Could you check a few things on this model? Use its own coordinates, in mm. A direction names the side the tool comes from. Give positions to 0.01 mm unless a question says otherwise; leave off trailing zeros. Loops run counter-clockwise (first coordinate to the right, second up) from the corner with the lowest first, then second, coordinate; pieces in that order, holes last. Notation, with made-up numbers: (-28.75, 6) -> (6.25, 6) arc R21 ccw to (6.25, 30) -> close; hole circle Ø11 at (-16.75, -19.5). An arc over 180 degrees is marked (long way). Write item = value, one per line. Start each with the question number.
1) I need wall thicknesses on probe 1 along Z at (x, y) = (-7, 22.75); probe 2 along Z at (x, y) = (-9.25, 22.75); probe 3 along Y at (x, z) = (-6.25, -6.5). Which ranges of each line are inside material? Lowest first, please. Write a range as from..to.
2) I want a section at B-B (z = -5.25). List the corners of the cut face in (x, y) for me.
3) I want a section at A-A (y = 22). List the corners of the cut face in (x, z) for me.
4) If we mould it in two halves opening along Z, with no side actions, what happens to faces 4 (the face through (-8, 12, 0)), 5 (the face through (-8, 12, -27.62)), 6 (the face through (-15, 12, -14)), 7 (the face through (-8, 3, -21))? For each: +Z half, -Z half, draft (parallel to the pull), parting line (faces both ways), or undercut.
5) I'm going to push flat-ended pins straight in: pin 1 Ø1.2 at (x, z) = (-7.5, -6.5) entering from -Y; pin 2 Ø1.2 at (x, z) = (-6.5, -7.5) entering from +Y. Where does each tip first touch, or does it pass through?
6) On a 3-axis mill with a long thin cutter (end or side, diameter ignored), from which of +Z, -Z, +X, -X, +Y, -Y can I reach the whole of each face in a straight line? I mean faces 1 (the face through (-8, 21.52, -21)), 2 (the face through (-8, 3, -7)), 3 (the face through (-8, 0, -14)). Say none if no direction works.
from build123d import *

# Parameters (mm, degrees)
ESQUISSE1_W             = 15
ESQUISSE1_H             = 24.52
BOSS_EXTRU_1_DEPTH      = 27.62
ENL_V_MAT_EXTRU_1_DEPTH = 3
ENL_V_MAT_EXTRU_2_DEPTH = 3


with BuildPart() as part:
    # Esquisse1 → Boss.-Extru.1 (new body)
    with BuildSketch(Plane.XY):
        with Locations((-7.5, 12.26)):
            Rectangle(ESQUISSE1_W, ESQUISSE1_H)
    extrude(amount=-BOSS_EXTRU_1_DEPTH)

    # Esquisse2 → Enlèv. mat.-Extru.1 (cut)
    with BuildSketch(Plane(origin=(0, 24.52, 0), x_dir=(1, 0, 0), z_dir=(0, 1, 0))):
        with BuildLine():
            ThreePointArc((-7.5, 23.0875), (-9.5, 21.0875), (-7.5, 19.0875))
            Line((-7.5, 19.0875), (-7.5, 23.0875))
        make_face()
        with BuildLine():
            Line((-7.5, 23.0875), (-7.5, 19.0875))
            ThreePointArc((-7.5, 19.0875), (-6.085786438, 19.673286438), (-5.5, 21.0875))
            ThreePointArc((-5.5, 21.0875), (-6.085786438, 22.501713562), (-7.5, 23.0875))
        make_face()
        with BuildLine():
            ThreePointArc((-5.5, 8.0225), (-6.085786438, 9.436713562), (-7.5, 10.0225))
            Line((-7.5, 10.0225), (-7.5, 6.0225))
            ThreePointArc((-7.5, 6.0225), (-6.085786438, 6.608286438), (-5.5, 8.0225))
        make_face()
        with BuildLine():
            Line((-7.5, 6.0225), (-7.5, 10.0225))
            ThreePointArc((-7.5, 10.0225), (-9.5, 8.0225), (-7.5, 6.0225))
        make_face()
    extrude(amount=-ENL_V_MAT_EXTRU_1_DEPTH, mode=Mode.SUBTRACT)

    # Esquisse3 → Enlèv. mat.-Extru.2 (cut)
    with BuildSketch(Plane.XZ):
        with BuildLine():
            ThreePointArc((-7.5, -4.905), (-9.5, -6.905), (-7.5, -8.905))
            Line((-7.5, -8.905), (-7.5, -4.905))
        make_face()
        with BuildLine():
            Line((-7.5, -4.905), (-7.5, -8.905))
            ThreePointArc((-7.5, -8.905), (-6.085786438, -8.319213562), (-5.5, -6.905))
            ThreePointArc((-5.5, -6.905), (-6.085786438, -5.490786438), (-7.5, -4.905))
        make_face()
        with BuildLine():
            ThreePointArc((-5.5, -20.715), (-6.085786438, -19.300786438), (-7.5, -18.715))
            Line((-7.5, -18.715), (-7.5, -22.715))
            ThreePointArc((-7.5, -22.715), (-6.085786438, -22.129213562), (-5.5, -20.715))
        make_face()
        with BuildLine():
            Line((-7.5, -22.715), (-7.5, -18.715))
            ThreePointArc((-7.5, -18.715), (-9.5, -20.715), (-7.5, -22.715))
        make_face()
    extrude(amount=-ENL_V_MAT_EXTRU_2_DEPTH, mode=Mode.SUBTRACT)


solid = part.part
Answer list:
q1.probe_1 = -27.62..-23.02, -19.15..-9.96, -6.09..0
q1.probe_2 = -27.62..-22.06, -20.12..-8.99, -7.05..0
q1.probe_3 = 3..21.52
q2.outline = (-15, 0) -> (-8.62, 0) -> (-8.62, 3) -> (-6.38, 3) -> (-6.38, 0) -> (0, 0) -> (0, 24.52) -> (-15, 24.52) -> close
q3.outline = (-15, -27.62) -> (0, -27.62) -> (0, 0) -> (-15, 0) -> close; hole circle Ø4 at (-7.5, -21.09); hole circle Ø4 at (-7.5, -8.02)
q4.face_4 = +Z half
q4.face_5 = -Z half
q4.face_6 = draft
q4.face_7 = undercut
q5.pin_1 = 3
q5.pin_2 = 21.52
q6.face_1 = +Y
q6.face_2 = -Y
q6.face_3 = +Z, -Z, +X, -X, -Y
